```python
from build123d import *

# Parameters (mm, degrees)
SKETCH1_R           = 10
BOSS_EXTRUDE1_DEPTH = 3
SKETCH2_R           = 2.55
CUT_EXTRUDE1_DEPTH  = 2.6
FILLET1_R           = 0.4
BOSS_EXTRUDE2_START = 1.4
SKETCH3_R           = 4.5
SKETCH3_R_2         = 2.55
BOSS_EXTRUDE2_DEPTH = 1.4
FILLET2_R           = 0.8
FILLET3_R           = 0.8


with BuildPart() as part:
    # Sketch1 → Boss-Extrude1 (new body)
    with BuildSketch(Plane(origin=(0, 0, 0), x_dir=(1, 0, 0), z_dir=(0, 1, 0))):
        with Locations(Location((0, 0, 0), (0, 0, 270))):
            Circle(SKETCH1_R)
    extrude(amount=BOSS_EXTRUDE1_DEPTH)

    # Sketch2 → Cut-Extrude1 (cut)
    with BuildSketch(Plane(origin=(0, 3, 0), x_dir=(1, 0, 0), z_dir=(0, 1, 0))):
        with Locations(Location((0, 0, 0), (0, 0, 270))):
            Circle(SKETCH2_R)
    extrude(amount=-CUT_EXTRUDE1_DEPTH, mode=Mode.SUBTRACT)

    # Fillet1
    fillet1_edges = [part.edges().sort_by_distance(p)[0] for p in [
        (0, 0, -10),
        (0, 3, -10),
    ]]
    fillet(fillet1_edges, radius=FILLET1_R)

    # Sketch3 → Boss-Extrude2 (add)
    with BuildSketch(Plane(origin=(0, 3, 0), x_dir=(1, 0, 0), z_dir=(0, 1, 0)).offset(BOSS_EXTRUDE2_START)):
        with Locations(Location((0, 0, 0), (0, 0, 270))):
            Circle(SKETCH3_R)
        with Locations(Location((0, 0, 0), (0, 0, 270))):
            Circle(SKETCH3_R_2, mode=Mode.SUBTRACT)
    extrude(amount=-BOSS_EXTRUDE2_DEPTH)

    # Fillet2
    fillet2_edges = [part.edges().sort_by_distance(p)[0] for p in [
        (0, 3, -4.5),
    ]]
    fillet(fillet2_edges, radius=FILLET2_R)

    # Fillet3
    fillet3_edges = [part.edges().sort_by_distance(p)[0] for p in [
        (0, 4.4, -4.5),
    ]]
    fillet(fillet3_edges, radius=FILLET3_R)


solid = part.part
```
Design review of the part built by this model. Coordinates are the model's own, in mm. A direction names the side the tool comes from. Give positions to 0.01 mm unless a question says otherwise; leave off trailing zeros. Return JSON: item names as keys, results as strings. Group by question number.
(1) Insertion check: pin 1 (1.5 mm diameter, centred on x = 1, z = 0.5, fed in from +Y); pin 2 (1 mm diameter, centred on x = -2, y = 3, fed in from -Z). Each pin has a flat end and moves straight along its axis. Give the tip position at first contact, or say it passes through.
(2) Machinability: for faces 1 (the flat face through (-4, 3, 4)), 2 (the flat face through (-3, 4.4, 0)), which of the approach directions +Z, -Z, +X, -X, +Y, -Y give a long, thin tool a straight path to every point of the face, cutting with its end or side? Answer none if there is none.
(3) Mouldability with a two-part tool opening along Z and no side actions: class faces 3 (the flat face through (0, 0, 0)), 4 (the flat face through (0, 0.4, 0)), 5 (the cylindrical face through (-9.76, 1.48, -2.17)) as +Z half, -Z half, draft (parallel to the pull), parting line (faces both ways), or undercut.
(4) To check wall thickness, follow probe 1 along X at (y, z) = (1.3, 0); probe 2 along Y at (x, z) = (-3, 4.5); probe 3 along Z at (x, y) = (-0.75, 2.7). State the ranges of each line that lie inside material, in increasing order.
Reported:
{
 "1": {"pin 1": "stops at y = 0.4", "pin 2": "stops at z = -9.86"},
 "2": {"face 1": "+Y", "face 2": "+Z, -Z, +X, -X, +Y"},
 "3": {"face 3": "draft", "face 4": "undercut", "face 5": "parting line"},
 "4": {"probe 1": "x = -10 to -2.55, 2.55 to 10", "probe 2": "y = 0 to 3", "probe 3": "z = -9.96 to -2.44, 2.44 to 9.96"}
}
